from build123d import *

# Parameters (mm, degrees)
SKETCH2_R          = 5
SKETCH2_R_2        = 4
CUT_EXTRUDE1_DEPTH = 30
SKETCH3_W          = 20.330301562
SKETCH3_H          = 41.442025473
SKETCH3_W_2        = 16.200064503
SKETCH3_H_2        = 44.818824912
CUT_EXTRUDE2_DEPTH = 20
SKETCH4_W          = 10
SKETCH4_H          = 24
CUT_EXTRUDE3_DEPTH = 20


with BuildPart() as part:
    # Sketch1 → Revolve1 (revolve)
    with BuildSketch(Plane(origin=(0, 0, 0), x_dir=(0, 0, -1), z_dir=(1, 0, 0))):
        with BuildLine():
            Line((-18, 0), (77, 0))
            ThreePointArc((77, 0), (73.485281374, 8.485281374), (65, 12))
            Line((65, 12), (0, 18))
            ThreePointArc((0, 18), (-12.727922061, 12.727922061), (-18, 0))
        make_face()
    revolve(axis=Axis((0, 0, 43.473022029), (0, 0, -1)))

    # Sketch2 → Cut-Extrude1 (cut, symmetric)
    with BuildSketch(Plane(origin=(0, 0, 0), x_dir=(0, 0, -1), z_dir=(1, 0, 0))):
        with Locations(Location((0, 0, 0), (0, 0, 270))):
            Circle(SKETCH2_R)
        with Locations(Location((65, 0, 0), (0, 0, 90))):
            Circle(SKETCH2_R_2)
    extrude(amount=CUT_EXTRUDE1_DEPTH, both=True, mode=Mode.SUBTRACT)

    # Sketch3 → Cut-Extrude2 (cut, symmetric)
    with BuildSketch(Plane(origin=(0, 0, 0), x_dir=(1, 0, 0), z_dir=(0, 1, 0))):
        with Locations((-16.165150781, -0.721012737)):
            Rectangle(SKETCH3_W, SKETCH3_H)
        with Locations((14.100032252, -2.409412456)):
            Rectangle(SKETCH3_W_2, SKETCH3_H_2)
    extrude(amount=CUT_EXTRUDE2_DEPTH, both=True, mode=Mode.SUBTRACT)

    # Sketch4 → Cut-Extrude3 (cut, symmetric)
    with BuildSketch(Plane(origin=(0, 0, 0), x_dir=(1, 0, 0), z_dir=(0, 1, 0))):
        with Locations((0, 65)):
            Rectangle(SKETCH4_W, SKETCH4_H)
    extrude(amount=CUT_EXTRUDE3_DEPTH, both=True, mode=Mode.SUBTRACT)


solid = part.part
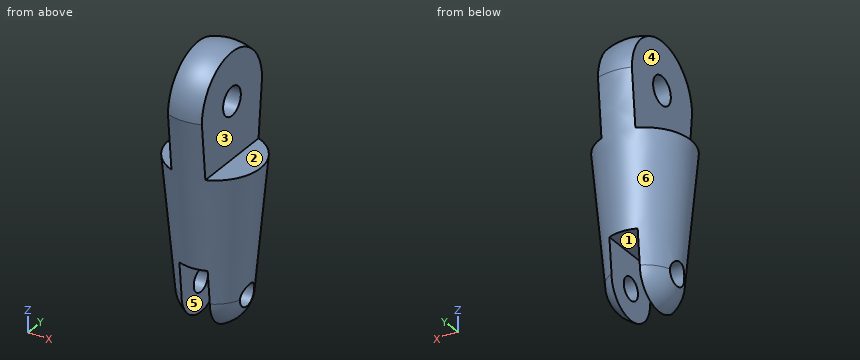
Part model, mm, in its own coordinate system. Face numbers are marked on the shaded views. A direction names the side the tool comes from. Round coordinates to 2 decimals unless told otherwise and drop trailing zeros. Order: outer loops, then holes, each group sorted by start corner. A loop starts at its lowest first (then second) coordinate and runs counter-clockwise, first axis right, second up. Notation, with made-up numbers: (73.5, -3) -> (78.5, -3) arc R21 ccw to (78.5, 6) -> close; hole circle Ø10 at (18, 70). An arc over 180 degrees is marked (long way). Put each result on its own line as item: value.
Q1. Band-saw the part on C-C (z = -27). Give the cut face in (x, y).
From the geometry:
outline: circle Ø31.02 at (0, 0)
Q2. Band-saw the part on A-A (z = 4). Give the cut face in (x, y).
From the geometry:
outline: (-6, -16.49) arc R17.55 ccw to (6, -16.49) -> (6, -3) -> (-6, -3) -> close; (-6, 3) -> (6, 3) -> (6, 16.49) arc R17.55 ccw to (-6, 16.49) -> close
Q3. Pin check, flat tips, straight feed: pin 1 Ø2 at (y, z) = (-6, -41.5) entering from -X; pin 2 Ø5 at (x, y) = (11, 1.5) entering from +Z; pin 3 Ø8 at (x, z) = (-3, 4) entering from -Y; pin 4 Ø9 at (y, z) = (0, 0) entering from -X. Stop position of each tip, or through.
From the geometry:
pin 1: stops at x = -13.27
pin 2: stops at z = -20
pin 3: stops at y = -17.97
pin 4: passes through
Q4. Band-saw the part on B-B (y = -2). State how many separate pieces and enclosed holes the cut face has, and give its area (3 significant figures).
From the geometry:
separate pieces: 4
enclosed holes: 0
area: 1,490 mm2
Q5. Pull direction X, two halves, no side cores. Call the marked faces 1, 2 and 3: pulls with the +X half, pulls with the -X half, needs draft (parallel to the pull), parting line crosses it, or undercut.
From the geometry:
face 1: undercut
face 2: needs draft
face 3: pulls with the +X half
Q6. Tool access for the marked faces 4, 5 and 6: list every direction of +Z, -Z, +X, -X, +Y, -Y with a clear straight run to the whole face (end or side of a thin tool).
From the geometry:
face 4: +Z, -X, +Y, -Y
face 5: -Z, +Y, -Y
face 6: -Z
Q7. Wall check: line 1 (X direction, y = 6.5, z = -53.5); line 2 (X direction, y = -14.5, z = -1); line 3 (Z direction, x = 3, y = 9.5). Give the ranges that are in metal, low to high. Write a range as [from, to].
From the geometry:
line 1: x = [-11.33, -5], [5, 11.33]
line 2: x = [-6, 6]
line 3: z = [-53, 14.99]
